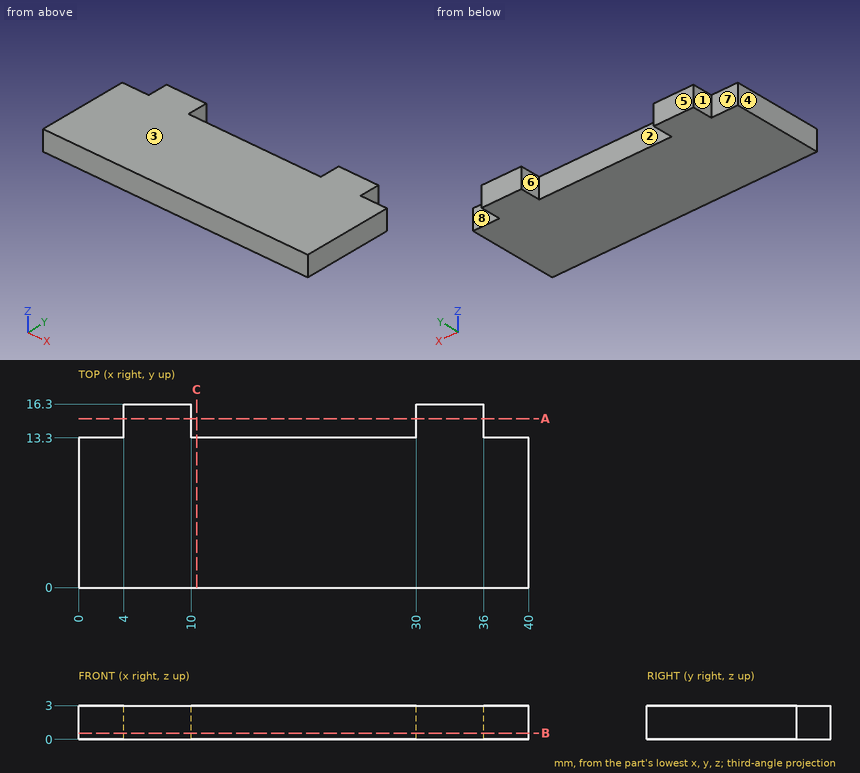
Could you check a few things on this drawing? It's one solid part, dimensions in mm from its lowest x, y, z. A direction names the side the tool comes from. Give positions to 0.01 mm unless a question says otherwise; leave off trailing zeros. Write each loop counter-clockwise with the first axis right and the second up, starting at its lowest first coordinate (ties: lowest second). Pieces come first, ordered by that corner, then holes. Notation, with made-up numbers: (85, 7) -> (107, 7) arc R24 ccw to (107, 27) -> close; hole circle Ø4 at (24.5, 6.25). An arc over 180 degrees is marked (long way). Write each question's results on one line, items separated by ' | '.
1. Will these pins go through, and if not, where does the flat tip stop? pin 1 Ø1.5 at (x, y) = (34.5, 3.5) entering from -Z; pin 2 Ø0.9 at (x, z) = (16.5, 1) entering from +Y; pin 3 Ø0.9 at (y, z) = (15, 1) entering from -X.
Check sheet entries:
pin 1: stops at z = 0 | pin 2: stops at y = 13.3 | pin 3: stops at x = 4
2. If we mould it in two halves opening along X, with no side actions, what happens to the marked faces 1, 2 and 3? For each: released by +X, released by -X, zero draft, split by the parting line, or undercut.
Check sheet entries:
face 1: released by -X | face 2: undercut | face 3: zero draft
3. I want a section at A-A, the plane y = 15. Write out the boundary of the cut face in (x, z), then the cut area to 3 significant figures.
Check sheet entries:
outline: (4, 0) -> (10, 0) -> (10, 3) -> (4, 3) -> close; (30, 0) -> (36, 0) -> (36, 3) -> (30, 3) -> close | area: 36.0 mm²
4. I want a section at B-B, the plane z = 0.55. Write out the boundary of the cut face in (x, y).
Check sheet entries:
outline: (0, 0) -> (40, 0) -> (40, 13.3) -> (36, 13.3) -> (36, 16.3) -> (30, 16.3) -> (30, 13.3) -> (10, 13.3) -> (10, 16.3) -> (4, 16.3) -> (4, 13.3) -> (0, 13.3) -> close
5. I need wall thicknesses on L1, parallel to X at y = 15.5, z = 2.45; L2, parallel to Y at x = 19.5, z = 1.95. Which ranges of each line are inside material? Lowest first, please.
Check sheet entries:
L1: x = 4 to 10, 30 to 36 | L2: y = 0 to 13.3
6. I want a section at C-C, the plane x = 10.5. Write out the boundary of the cut face in (y, z).
Check sheet entries:
outline: (0, 0) -> (13.3, 0) -> (13.3, 3) -> (0, 3) -> close
7. On a 3-axis mill with a long thin cutter (end or side, diameter ignored), from which of +Z, -Z, +X, -X, +Y, -Y can I reach the whole of each face in a straight line? I mean the marked faces 4, 5, 6, 7 and 8. Say none if no direction works.
Check sheet entries:
face 4: +Z, -Z, -X, +Y, -Y | face 5: +Z, -Z, +X, -X, +Y | face 6: +Z, -Z, +Y | face 7: +Z, -Z, -X, +Y | face 8: +Z, -Z, +X, +Y
